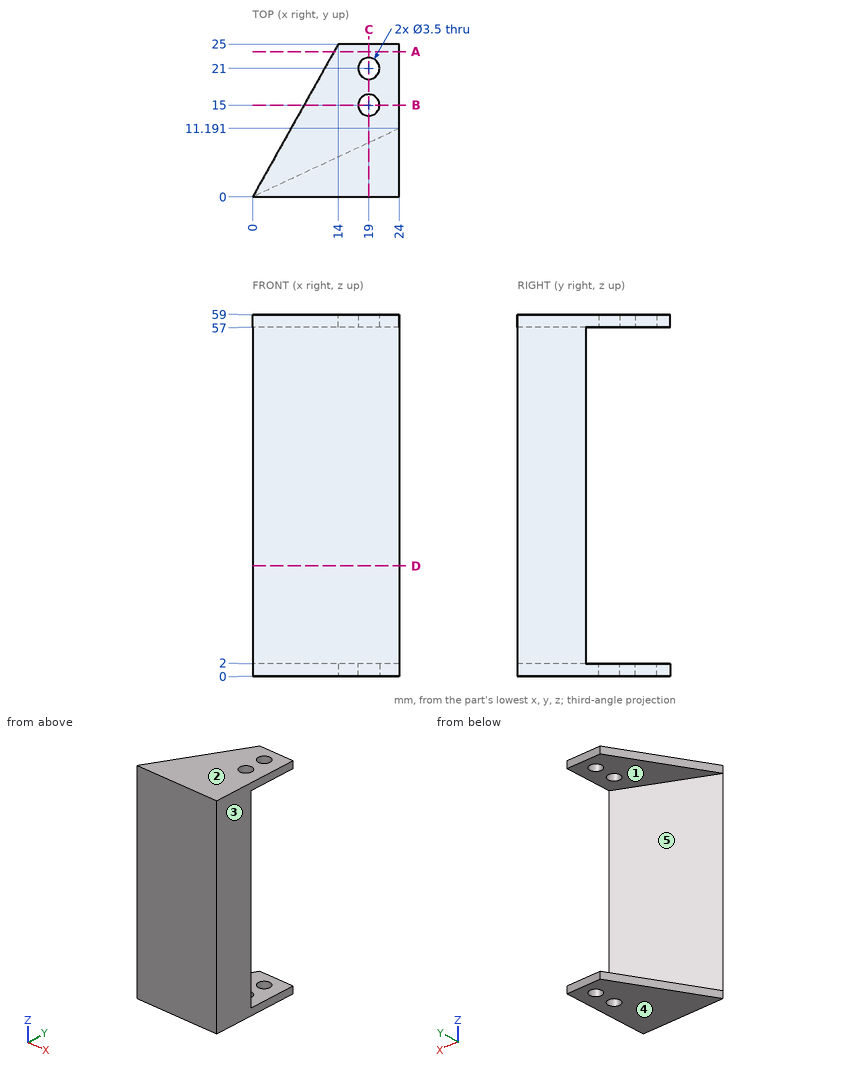
Study the drawing (mm; zero at the part's minimum x, y, z) and answer. A direction names the side the tool comes from. Give positions to 0.01 mm unless a question says otherwise; leave off trailing zeros. Write each loop counter-clockwise with the first axis right and the second up, starting at its lowest first coordinate (ties: lowest second). Pieces come first, ordered by that corner, then holes. Notation, with made-up numbers: (-7.5, 26.25) - (17.5, 26.25) arc R25 cw to (17.5, 61.25) - close; hole circle Ø11 at (-35.75, 24.5). An arc over 180 degrees is marked (long way). Use a Markdown table: item, result.
1. For a pull along X with two mould halves and no side action, classify the marked faces 3, 4 and 5 as released by +X, released by -X, zero draft, split by the parting line, or undercut.
Values follow:
| item | result |
|---|---|
| face 3 | released by +X |
| face 4 | zero draft |
| face 5 | released by -X |
2. Section A-A on y = 23.75 is taken. Write down the section's boundary in (x, z).
Values follow:
| item | result |
|---|---|
| outline | (13.3, 0) - (24, 0) - (24, 2) - (13.3, 2) - close; (13.3, 57) - (24, 57) - (24, 59) - (13.3, 59) - close |
3. Section B-B on y = 15 is taken. Write down the section's boundary in (x, z), plus the area to 3 significant figures.
Values follow:
| item | result |
|---|---|
| outline | (8.4, 0) - (17.25, 0) - (17.25, 2) - (8.4, 2) - close; (8.4, 57) - (17.25, 57) - (17.25, 59) - (8.4, 59) - close; (20.75, 0) - (24, 0) - (24, 2) - (20.75, 2) - close; (20.75, 57) - (24, 57) - (24, 59) - (20.75, 59) - close |
| area | 48.4 mm² |
4. Each of these flat-tipped pins is pushed along its axis until it touches: P1, Ø5, axis at x = 14.5, y = 19.5, coming from the -Z side; P2, Ø8, axis at y = 5.5, z = 8, coming from the -X side (1 decimal); P3, Ø2, axis at x = 19, y = 21, coming from the +Z side. Where does it stop, or does it pass through?
Values follow:
| item | result |
|---|---|
| P1 | stops at z = 0 |
| P2 | stops at x = 3.2 |
| P3 | passes through |
5. A tool of negligible diameter and unlimited length cuts with its end or side. For the marked faces 1 and 2, from which of +Z, -Z, +X, -X, +Y, -Y can it reach the whole face along a straight path? Write none if from no direction.
Values follow:
| item | result |
|---|---|
| face 1 | -X, +Y |
| face 2 | +Z, +X, -X, +Y, -Y |
6. Find the intervals of material crossed by probe 1 along Y at (x, z) = (19, 58.5); probe 2 along Z at (x, y) = (22.5, 15.25); probe 3 along Y at (x, z) = (10.25, 18), in increasing order. Write a range as from..to.
Values follow:
| item | result |
|---|---|
| probe 1 | y = 0..13.25, 16.75..19.25, 22.75..25 |
| probe 2 | z = 0..2, 57..59 |
| probe 3 | y = 0..4.78 |
7. Section D-D on z = 18 is taken. Write down the section's boundary in (x, y).
Values follow:
| item | result |
|---|---|
| outline | (0, 0) - (24, 0) - (24, 11.19) - close |
8. Section C-C on x = 19 is taken. Write down the section's boundary in (y, z).
Values follow:
| item | result |
|---|---|
| outline | (0, 0) - (13.25, 0) - (13.25, 2) - (8.86, 2) - (8.86, 57) - (13.25, 57) - (13.25, 59) - (0, 59) - close; (16.75, 0) - (19.25, 0) - (19.25, 2) - (16.75, 2) - close; (16.75, 57) - (19.25, 57) - (19.25, 59) - (16.75, 59) - close; (22.75, 0) - (25, 0) - (25, 2) - (22.75, 2) - close; (22.75, 57) - (25, 57) - (25, 59) - (22.75, 59) - close |
